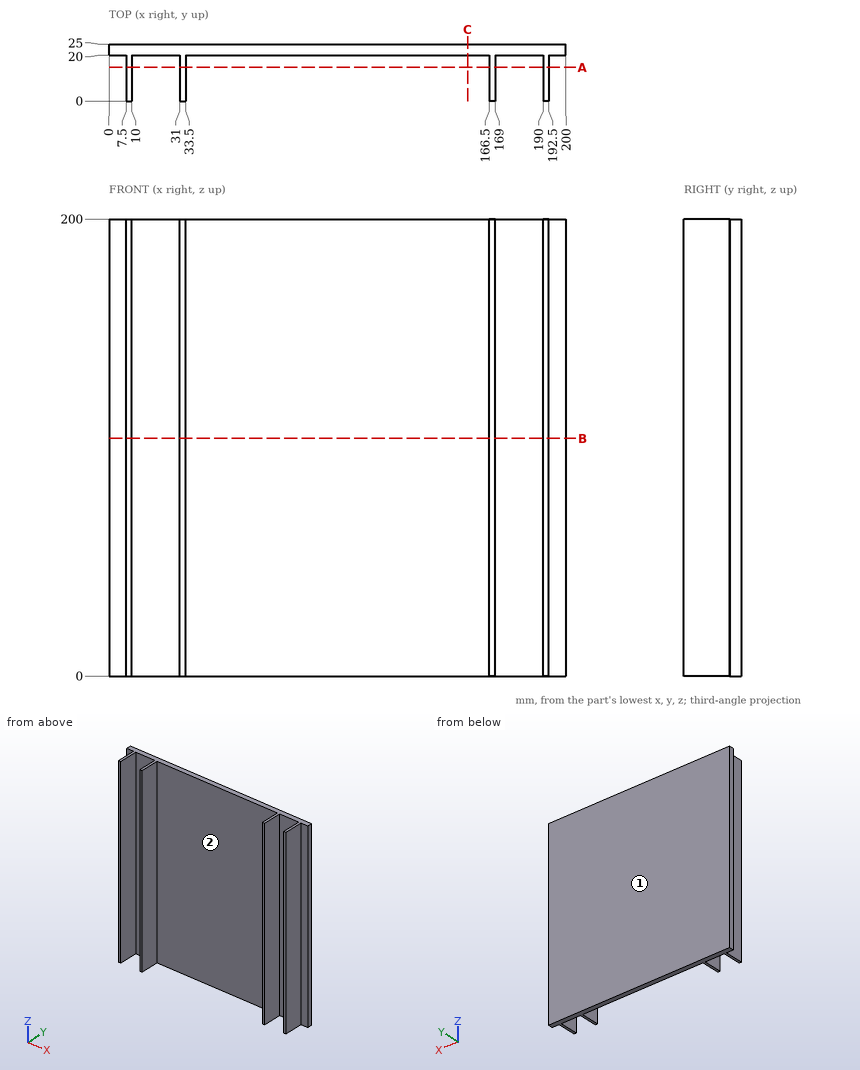
Geometry: see drawing. Coordinates: mm, zero at the bounding-box minimum. Coordinates: 2 decimals unless noted, no trailing zeros. Order: outer loops, then holes, each group sorted by start corner. A loop starts at its lowest first (then second) coordinate and runs counter-clockwise, first axis right, second up. Notation, with made-up numbers: (-34.5, -8.75) - (-12.5, -8.75) arc R18 ccw to (-12.5, -0.75) - close; hole circle Ø1 at (-11, 53). An arc over 180 degrees is marked (long way). Write each question's results on one line, items separated by ' | '.
1) Line query: line 1 (X direction, y = 17, z = 121.5); line 2 (Y direction, x = 134, z = 47.5). Output: solid intervals per line, ascending. Write a range as from..to.
Results list:
line 1: 7.5..10, 31..33.5, 166.5..169, 190..192.5 | line 2: 20..25
2) Pull-direction query (X, two-part tool) for the marked faces 1 and 2; classes: pulls with the +X half, pulls with the -X half, needs draft (parallel to the pull), parting line crosses it, or undercut.
Results list:
face 1: needs draft | face 2: undercut
3) Section C-C, the plane x = 157. Return loops of the section in (y, z).
Results list:
outline: (20, 0) - (25, 0) - (25, 200) - (20, 200) - close
4) Section A-A, the plane y = 14.75. Return loops of the section in (x, z), plus the area to 3 significant figures.
Results list:
outline: (7.5, 0) - (10, 0) - (10, 200) - (7.5, 200) - close; (31, 0) - (33.5, 0) - (33.5, 200) - (31, 200) - close; (166.5, 0) - (169, 0) - (169, 200) - (166.5, 200) - close; (190, 0) - (192.5, 0) - (192.5, 200) - (190, 200) - close | area: 2,000 mm^2
5) Pin query (flat end, axial travel): pin 1 (3 mm diameter, centred on y = 10, z = 94, fed in from -X); pin 2 (1 mm diameter, centred on x = 62, y = 22, fed in from -Z); pin 3 (10 mm diameter, centred on y = 14.5, z = 69, fed in from +X); pin 4 (12 mm diameter, centred on x = 176.5, z = 67, fed in from -Y). Return the tip coordinate at first contact, or that it passes through.
Results list:
pin 1: x = 7.5 | pin 2: z = 0 | pin 3: x = 192.5 | pin 4: y = 20
6) Section B-B, the plane z = 104. Return loops of the section in (x, y), plus the area to 3 significant figures.
Results list:
outline: (0, 20) - (7.5, 20) - (7.5, 0) - (10, 0) - (10, 20) - (31, 20) - (31, 0) - (33.5, 0) - (33.5, 20) - (166.5, 20) - (166.5, 0) - (169, 0) - (169, 20) - (190, 20) - (190, 0) - (192.5, 0) - (192.5, 20) - (200, 20) - (200, 25) - (0, 25) - close | area: 1,200 mm^2
